Build history of the part. All positions in model axes, mm. Round coordinates to 2 decimals unless told otherwise and drop trailing zeros. Order: outer loops, then holes, each group sorted by start corner. A loop starts at its lowest first (then second) coordinate and runs counter-clockwise, first axis right, second up. Notation, with made-up numbers: (34.5, 20.25) -> (89.5, 20.25) arc R12 ccw to (89.5, 30.25) -> close; hole circle Ø6 at (60.25, 54.5). An arc over 180 degrees is marked (long way). Write item = value, one per line.
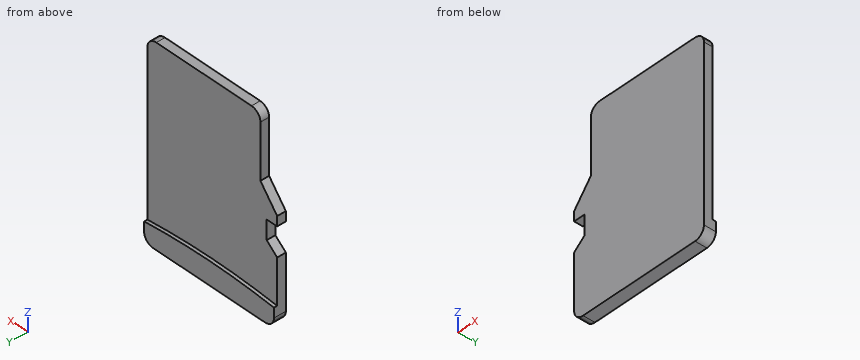
Autodesk Inventor part; units mm, degrees
ref_plane "YZ Plane" through (0, 0, 0) normal (1, 0, 0) x (0, 1, 0)
ref_plane "XZ Plane" through (0, 0, 0) normal (0, 1, 0) x (-1, 0, 0)
ref_plane "XY Plane" through (0, 0, 0) normal (0, 0, 1) x (1, 0, 0)
sketch "Sketch1" plane through (0, 0, 0) normal (0, 1, 0) x (-1, 0, 0)
  line L0 (-1.4224, 0) -> (-11.049, 0)
  line L1 (-11.049, 0) -> (-11.049, -14.986)
  line L2 (-11.049, -14.986) -> (0, -14.986)
  line L3 (0, -14.986) -> (0, -9.906)
  line L4 (0, -9.906) -> (-0.889, -9.144)
  line L5 (-0.889, -9.144) -> (-0.889, -7.62)
  line L6 (-0.889, -7.62) -> (0, -7.62)
  line L7 (0, -7.62) -> (0, -6.858)
  line L8 (0, -6.858) -> (-1.4224, -5.08)
  line L9 (-1.4224, -5.08) -> (-1.4224, 0)
  point P0 (0, 0)
  dimension "d0" = 14.986
  dimension "d1" = 11.049
  dimension "d2" = 9.6266
  dimension "d3" = 0.889
  dimension "d4" = 5.08
  dimension "d5" = 7.62
  dimension "d6" = 0.762
  dimension "d7" = 1.778
  dimension "d8" = 5.08
extrude "Extrusion1" add sketch "Sketch1" along normal blind 0.6858
fillet "Fillet1" radius 0.762 4 edges at (11.049, 0.3429, -14.986) (0, 0.3429, -14.986) (11.049, 0.3429, 0) (1.4224, 0.3429, 0)
sketch "Sketch2" plane through (0, 0.6858, 0) normal (0, 1, 0) x (1, 0, 0)
  arc A0 (1.4224, 0.762) -> (2.1844, 0) centre (2.1844, 0.762) ccw
  line L0 (2.1844, 0) -> (10.287, 0)
  arc A1 (10.287, 0) -> (11.049, 0.762) centre (10.287, 0.762) ccw
  line L1 (11.049, 0.762) -> (11.049, 14.224)
  arc A2 (11.049, 14.224) -> (10.287, 14.986) centre (10.287, 14.224) ccw
  line L2 (10.287, 14.986) -> (0.762, 14.986)
  arc A3 (0.762, 14.986) -> (0, 14.224) centre (0.762, 14.224) ccw
  line L3 (0, 14.224) -> (0, 9.906)
  line L4 (0, 9.906) -> (0.889, 9.144)
  line L5 (0.889, 9.144) -> (0.889, 7.62)
  line L6 (0.889, 7.62) -> (0, 7.62)
  line L7 (0, 7.62) -> (0, 6.858)
  line L8 (0, 6.858) -> (1.4224, 5.08)
  line L9 (1.4224, 5.08) -> (1.4224, 0.762)
  line L10 (0, 14.224) -> (0, 9.906)
  arc A4 (0, 13.462) -> (11.049, 13.462) centre (5.5245, 65.5585) ccw
  point P0 (0, 0)
  dimension "d12" = 1.524
  dimension "d13" = 1.8161
extrude "Extrusion2" add sketch "Sketch2" along normal blind 0.254 contours A4 L3 A3 L2 A2 L1
properties part number "MicroSD Card"
Q1. Cut at B-B, the plane x = 3.75. List the corners of the cut face in (y, z).
Check values:
outline = (0, -14.99) -> (0.94, -14.99) -> (0.94, -13.2) -> (0.69, -13.2) -> (0.69, 0) -> (0, 0) -> close
Q2. Probe probe 1 along X at (y, z) = (0.4, -9); probe 2 along Y at (x, z) = (4.25, -5); probe 3 along X at (y, z) = (0.1, -5). List the from-to ranges inside material, lowest first.
Check values:
probe_1 = 0.89 to 11.05
probe_2 = 0 to 0.69
probe_3 = 1.42 to 11.05
Q3. Cut at C-C, the plane z = -11. List the corners of the cut face in (x, y).
Check values:
outline = (0, 0) -> (11.05, 0) -> (11.05, 0.69) -> (0, 0.69) -> close
Q4. Cut at D-D, the plane x = 6.25. List the corners of the cut face in (y, z), and give its area (3 significant figures).
Check values:
outline = (0, -14.99) -> (0.94, -14.99) -> (0.94, -13.17) -> (0.69, -13.17) -> (0.69, 0) -> (0, 0) -> close
area = 10.7 mm²
Q5. Cut at A-A, the plane y = 0.3. List the corners of the cut face in (x, z).
Check values:
outline = (0, -14.22) arc R0.76 ccw to (0.76, -14.99) -> (10.29, -14.99) arc R0.76 ccw to (11.05, -14.22) -> (11.05, -0.76) arc R0.76 ccw to (10.29, 0) -> (2.18, 0) arc R0.76 ccw to (1.42, -0.76) -> (1.42, -5.08) -> (0, -6.86) -> (0, -7.62) -> (0.89, -7.62) -> (0.89, -9.14) -> (0, -9.91) -> close
Q6. Flat gauge pin, fed straight in: pin 1 (1.5 mm diameter, centred on x = 1.5, z = -6.5, fed in from +Y). Where does the tip first touch, or does it go through?
Check values:
pin_1 = 0.69
